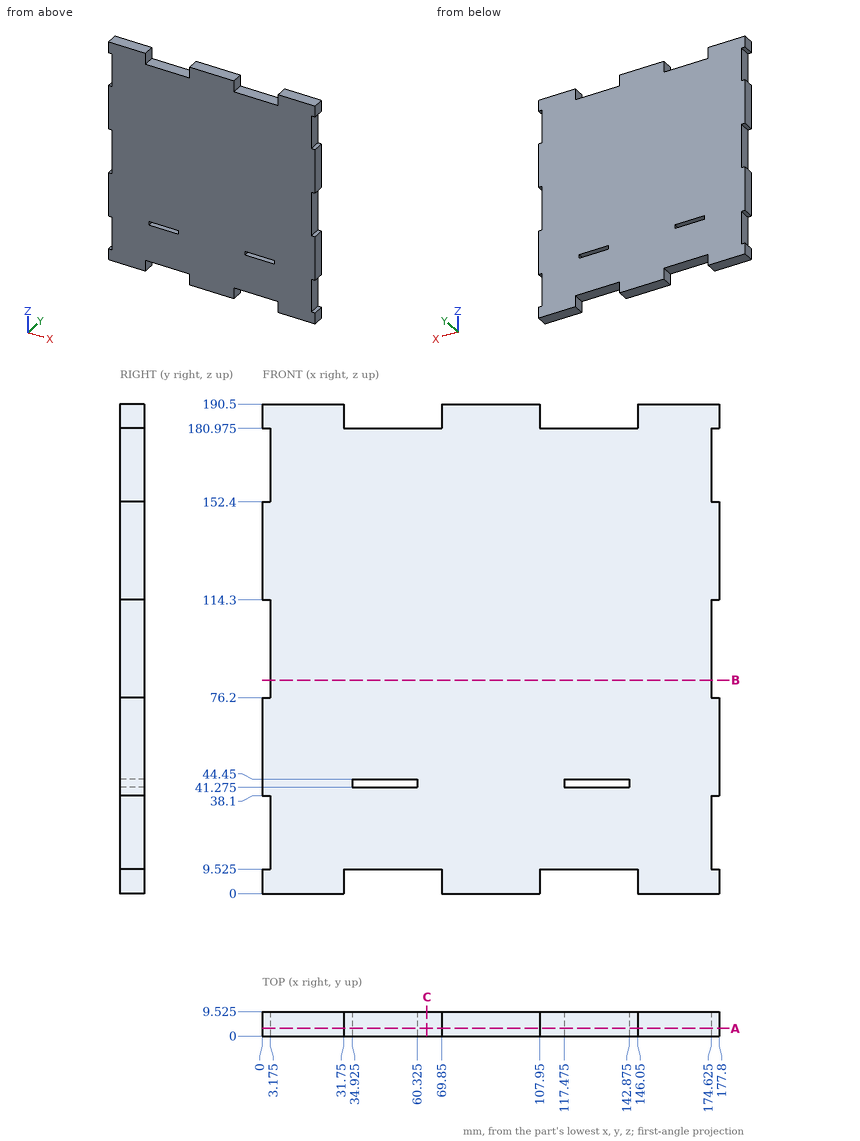
Job drawing, mm, ordinate dimensions from the low corner. One solid piece. Round coordinates to 2 decimals unless told otherwise and drop trailing zeros. Loops run counter-clockwise (first coordinate to the right, second up) from the corner with the lowest first, then second, coordinate; pieces in that order, holes last. Notation, with made-up numbers: (30, -1.75) -> (43, -1.75) arc R16 cw to (43, 29.25) -> close; hole circle Ø6 at (60.25, 87). An arc over 180 degrees is marked (long way). One line per item, written item: value. Start each with the question number.
Q1. Cut at B-B on z = 83. List the corners of the cut face in (x, y) (3 decimals), plus the area to 3 significant figures.
Q2. Drop a flat-ended pin along its axis: pin 1 Ø5 at (x, y) = (121.5, 7) entering from -Z (3 decimals). Give the stop position or say it passes through.
Q3. Cut at C-C on x = 64. List the corners of the cut face in (y, z) (3 decimals).
Q4. Probe line 1 along X through (y, z) = (9, 182.5); line 2 along Z through (x, y) = (125, 2) (3 decimals); line 3 along X through (y, z) = (6.5, 161.5) (3 decimals). List the from-to ranges inside material, lowest first.
Q5. Cut at A-A on y = 3. Count the separate pieces of the cut face and the enclosed holes in it, plus the area to 3 significant figures.
Computed:
1. outline: (3.175, 0) -> (174.625, 0) -> (174.625, 9.525) -> (3.175, 9.525) -> close
1. area: 1,630 mm²
2. pin 1: z = 9.525
3. outline: (0, 9.525) -> (9.525, 9.525) -> (9.525, 180.975) -> (0, 180.975) -> close
4. line 1: 0 to 31.75, 69.85 to 107.95, 146.05 to 177.8
4. line 2: 9.525 to 41.275, 44.45 to 180.975
4. line 3: 3.175 to 174.625
5. separate pieces: 1
5. enclosed holes: 2
5. area: 31,700 mm²
